The listing builds one solid part. Answer for the finished solid, in the listing's coordinates (mm). Face numbers are marked on the shaded views. Coordinates: 2 decimals unless noted, no trailing zeros. Order: outer loops, then holes, each group sorted by start corner. A loop starts at its lowest first (then second) coordinate and runs counter-clockwise, first axis right, second up. Notation, with made-up numbers: (-22, -38) -> (21, -38) arc R24 cw to (21, 0) -> close; hole circle Ø5 at (39, 53.5). An arc over 180 degrees is marked (long way). Return JSON: item names as keys, results as strings.
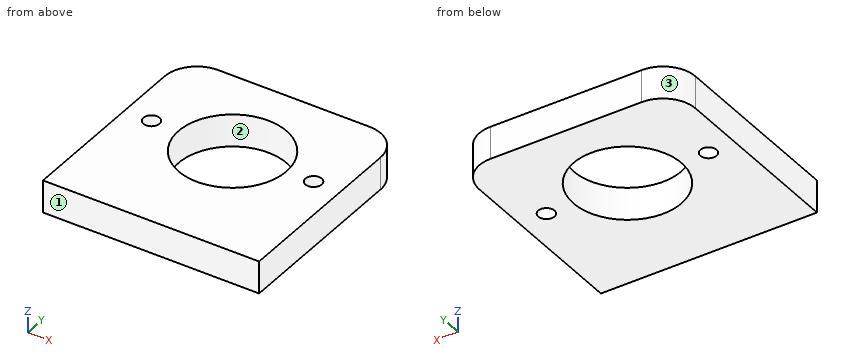
from build123d import *

# Parameters (mm, degrees)
SKETCH1_R           = 25
SKETCH1_R_2         = 3.75
BOSS_EXTRUDE1_DEPTH = 15


with BuildPart() as part:
    # Sketch1 → Boss-Extrude1 (new body)
    with BuildSketch(Plane.XY):
        with BuildLine():
            Line((-50, -57), (50, -57))
            Line((50, -57), (50, 28))
            ThreePointArc((50, 28), (45.606601718, 38.606601718), (35, 43))
            Line((35, 43), (-35, 43))
            ThreePointArc((-35, 43), (-45.606601718, 38.606601718), (-50, 28))
            Line((-50, 28), (-50, -57))
        make_face()
        Circle(SKETCH1_R, mode=Mode.SUBTRACT)
        with Locations((-37.5, 0)):
            Circle(SKETCH1_R_2, mode=Mode.SUBTRACT)
        with Locations(Location((37.5, 0, 0), (0, 0, 180))):
            Circle(SKETCH1_R_2, mode=Mode.SUBTRACT)
    extrude(amount=BOSS_EXTRUDE1_DEPTH)


solid = part.part
1. Consider line 1 (Y direction, x = 0, z = 6.5); line 2 (Y direction, x = -15, z = 12.5); line 3 (X direction, y = -14, z = 10.75). Determine where each line is inside the solid, lowest interval first. Write a range as from..to.
Answer block:
{"line 1": "y = -57..-25, 25..43", "line 2": "y = -57..-20, 20..43", "line 3": "x = -50..-20.71, 20.71..50"}
2. Determine the mould class of the marked faces 1, 2 and 3 for opening direction X: pulls with the +X half, pulls with the -X half, needs draft (parallel to the pull), parting line crosses it, or undercut.
Answer block:
{"face 1": "needs draft", "face 2": "undercut", "face 3": "pulls with the -X half"}
3. The part is cut by section B-B on x = 0. Give the vertices of the cut face in (y, z), and give its area (3 significant figures).
Answer block:
{"outline": "(-57, 0) -> (-25, 0) -> (-25, 15) -> (-57, 15) -> close; (25, 0) -> (43, 0) -> (43, 15) -> (25, 15) -> close", "area": "750 mm2"}
4. Each of these flat-tipped pins is pushed along its axis until it touches: pin 1 Ø12 at (x, y) = (13.5, 32) entering from -Z; pin 2 Ø6 at (x, y) = (-37.5, 0) entering from -Z. Where does it stop, or does it pass through?
Answer block:
{"pin 1": "stops at z = 0", "pin 2": "passes through"}
5. The part is cut by section C-C on z = 8.5. Give the vertices of the cut face in (x, y).
Answer block:
{"outline": "(-50, -57) -> (50, -57) -> (50, 28) arc R15 ccw to (35, 43) -> (-35, 43) arc R15 ccw to (-50, 28) -> close; hole circle Ø7.5 at (-37.5, 0); hole circle Ø50 at (0, 0); hole circle Ø7.5 at (37.5, 0)"}
6. The part is cut by section D-D on x = 15.5. Give the vertices of the cut face in (y, z), and give its area (3 significant figures).
Answer block:
{"outline": "(-57, 0) -> (-19.62, 0) -> (-19.62, 15) -> (-57, 15) -> close; (19.62, 0) -> (43, 0) -> (43, 15) -> (19.62, 15) -> close", "area": "912 mm2"}
7. The part is cut by section A-A on y = 0. Give the vertices of the cut face in (x, z), and give its area (3 significant figures).
Answer block:
{"outline": "(-50, 0) -> (-41.25, 0) -> (-41.25, 15) -> (-50, 15) -> close; (-33.75, 0) -> (-25, 0) -> (-25, 15) -> (-33.75, 15) -> close; (25, 0) -> (33.75, 0) -> (33.75, 15) -> (25, 15) -> close; (41.25, 0) -> (50, 0) -> (50, 15) -> (41.25, 15) -> close", "area": "525 mm2"}
